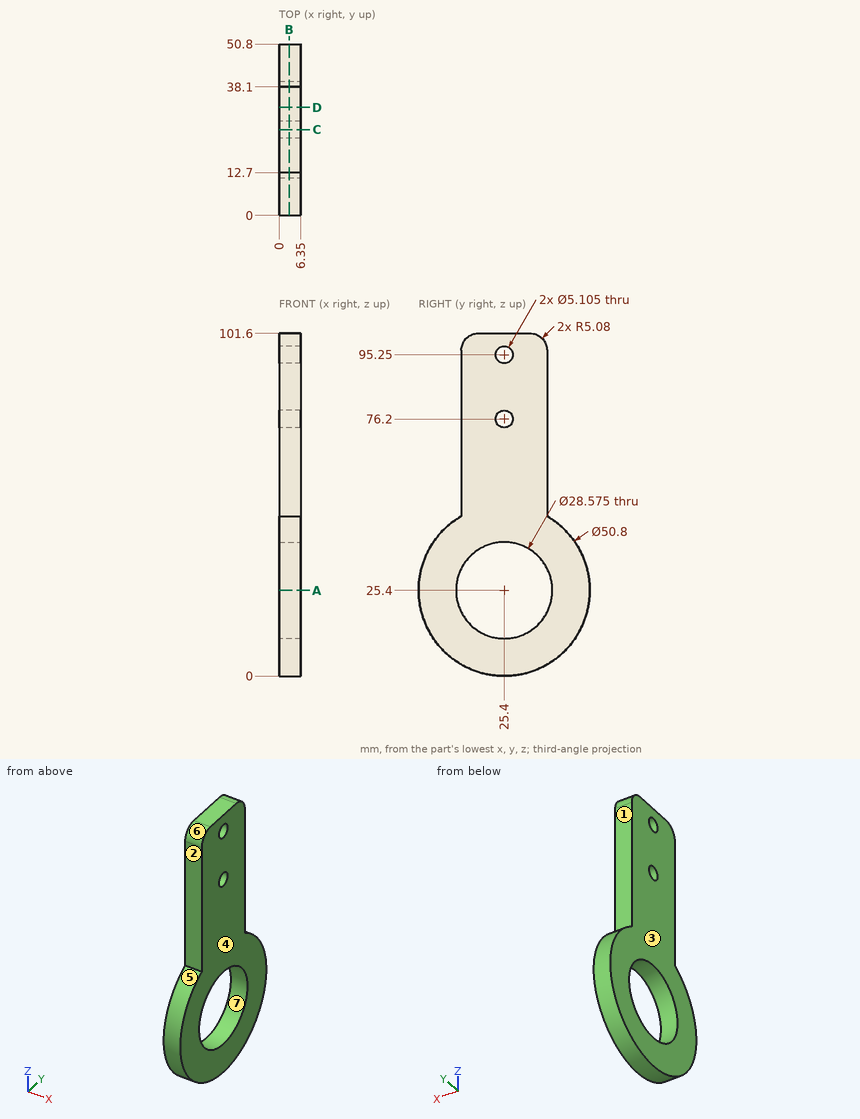
Job drawing, mm, ordinate dimensions from the low corner. One solid piece. A direction names the side the tool comes from. Round coordinates to 2 decimals unless told otherwise and drop trailing zeros. Order: outer loops, then holes, each group sorted by start corner. A loop starts at its lowest first (then second) coordinate and runs counter-clockwise, first axis right, second up. Notation, with made-up numbers: M 32,54.5 L 37,54.5 A18 cw 37,83.5 Z; hole C 34.25,16.25 d7. An arc over 180 degrees is marked long. Write each question's results on one line, items separated by ' | '. Start each with the question number.
(1) Two-plate mould, pull along Y, no slides. Class the marked faces 4, 5, 6 and 7: pulls with the +Y half, pulls with the -Y half, needs draft (parallel to the pull), parting line crosses it, or undercut.
(2) Which spindle directions (+Z, -Z, +X, -X, +Y, -Y) get a long thin tool onto all of the face, cutting with end or side? Do the marked faces 1, 2 and 3. Say none if no direction does.
(3) Saw through at D-D, the plane y = 32. Give the cut face in (x, z).
(4) Probe probe 1 along Y at (x, z) = (2, 76.2); probe 2 along Y at (x, z) = (0.5, 25.5); probe 3 along Z at (x, y) = (4.5, 24.5) (1 decimal). List the from-to ranges inside material, lowest first. Write a range as from..to.
(5) Saw through at A-A, the plane z = 25.4. Give the cut face in (x, y), then the cut area to 3 significant figures.
(6) Drop flat-ended pins along their axis: pin 1 (12 mm diameter, centred on y = 39, z = 33, fed in from -X); pin 2 (2 mm diameter, centred on x = 5, y = 24, fed in from -Z); pin 3 (2 mm diameter, centred on x = 2, z = 69, fed in from +Y). Give the stop position or say it passes through.
(7) Saw through at B-B, the plane x = 3. State how many separate pieces and enclosed holes the cut face has, then the cut area to 3 significant figures.
(8) Saw through at C-C, the plane y = 25.4. Give the cut face in (x, z).
Established:
1) face 4: needs draft | face 5: parting line crosses it | face 6: pulls with the -Y half | face 7: undercut
2) face 1: +Z, +X, -X, +Y | face 2: +Z, +X, -X, -Y | face 3: +Z, -Z, -X, +Y, -Y
3) outline: M 0,0.87 L 6.35,0.87 L 6.35,12.73 L 0,12.73 Z; M 0,38.07 L 6.35,38.07 L 6.35,101.6 L 0,101.6 Z
4) probe 1: y = 12.7..22.85, 27.95..38.1 | probe 2: y = 0..11.11, 39.69..50.8 | probe 3: z = 0..11.1, 39.7..73.8, 78.6..92.9, 97.6..101.6
5) outline: M 0,0 L 6.35,0 L 6.35,11.11 L 0,11.11 Z; M 0,39.69 L 6.35,39.69 L 6.35,50.8 L 0,50.8 Z | area: 141 mm^2
6) pin 1: stops at x = 0 | pin 2: stops at z = 0 | pin 3: stops at y = 38.1
7) separate pieces: 1 | enclosed holes: 3 | area: 2,650 mm^2
8) outline: M 0,0 L 6.35,0 L 6.35,11.11 L 0,11.11 Z; M 0,39.69 L 6.35,39.69 L 6.35,73.65 L 0,73.65 Z; M 0,78.75 L 6.35,78.75 L 6.35,92.7 L 0,92.7 Z; M 0,97.8 L 6.35,97.8 L 6.35,101.6 L 0,101.6 Z
